Work out the finished part from the listing and answer in its coordinate system (mm). Give positions to 0.01 mm unless a question says otherwise; leave off trailing zeros. Write each loop counter-clockwise with the first axis right and the second up, starting at its lowest first coordinate (ties: lowest second). Pieces come first, ordered by that corner, then holes. Notation, with made-up numbers: (8, -16.5) -> (56, -16.5) arc R27 ccw to (56, 13.5) -> close; hole circle Ø1 at (22, 64). An arc over 180 degrees is marked (long way). Write item = value, one per line. Start each with the question number.
from build123d import *

# Parameters (mm, degrees)
F1_DEPTH = 40
F2_DEPTH = 40
F3_R     = 5


with BuildPart() as f1:
    # F0 (on Top) → F1 (new body)
    with BuildSketch(Plane.XY):
        with BuildLine():
            Line((72.5, 131.3154598667), (72.5, 0))
            ThreePointArc((72.5, 0), (0, -72.5), (-72.5, 0))
            Line((-72.5, 0), (-72.5, 131.3154598667))
            ThreePointArc((-72.5, 131.3154598667), (-131.4940701743, 72.1755464751), (-149.7084414814, -9.3478633504))
            ThreePointArc((-149.7084414814, -9.3478633504), (-138.3891727392, -57.8656795395), (-111.803398875, -100))
            Line((-111.803398875, -100), (0, -100))
            Line((0, -100), (0, -150))
            ThreePointArc((0, -150), (106.066017178, -106.066017178), (150, 0))
            ThreePointArc((150, 0), (129.1801068276, 76.2397534099), (72.5, 131.3154598667))
        make_face()
        with BuildLine():
            ThreePointArc((-72.5, 0), (0, 72.5), (72.5, 0))
            Line((72.5, 0), (72.5, 131.3154598667))
            ThreePointArc((72.5, 131.3154598667), (0, 150), (-72.5, 131.3154598667))
            Line((-72.5, 131.3154598667), (-72.5, 0))
        make_face()
        with BuildLine():
            ThreePointArc((-111.803398875, -100), (-138.3891727392, -57.8656795395), (-149.7084414814, -9.3478633504))
            ThreePointArc((-149.7084414814, -9.3478633504), (-236.0979616676, -71.7417201282), (-338.8482034206, -100))
            Line((-338.8482034206, -100), (-111.803398875, -100))
        make_face()
        with BuildLine():
            Line((-750, -150), (0, -150))
            ThreePointArc((0, -150), (-61.2372435696, -136.9306393763), (-111.803398875, -100))
            Line((-111.803398875, -100), (-338.8482034206, -100))
            Line((-338.8482034206, -100), (-750, -100))
            Line((-750, -100), (-750, -150))
        make_face()
        with BuildLine():
            ThreePointArc((-111.803398875, -100), (-61.2372435696, -136.9306393763), (0, -150))
            Line((0, -150), (0, -100))
            Line((0, -100), (-111.803398875, -100))
        make_face()
    extrude(amount=F1_DEPTH)

    # F0 (on Top) → F2 (cut)
    with BuildSketch(Plane.XY):
        with BuildLine():
            ThreePointArc((-72.5, 0), (0, 72.5), (72.5, 0))
            Line((72.5, 0), (72.5, 131.3154598667))
            ThreePointArc((72.5, 131.3154598667), (0, 150), (-72.5, 131.3154598667))
            Line((-72.5, 131.3154598667), (-72.5, 0))
        make_face()
    extrude(amount=F2_DEPTH, mode=Mode.SUBTRACT)

    # F3
    f3_edges = [f1.edges().sort_by_distance(p)[0] for p in [
        (-750, -150, 20),
        (-72.5, 131.31546, 20),
        (72.5, 131.31546, 20),
        (-750, -100, 20),
    ]]
    fillet(f3_edges, radius=F3_R)


solid = f1.part
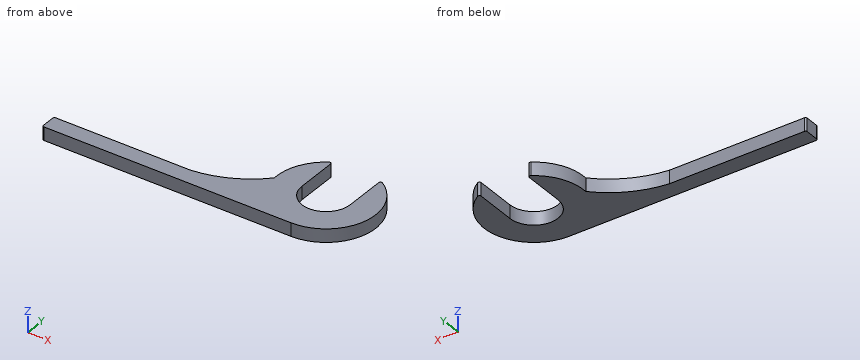
(1) Find the intervals of material crossed by line 1 along X through (y, z) = (3, 11.5); line 2 along X through (y, z) = (7.5, 27.5); line 3 along Y through (x, z) = (-523.5, 22), in increasing order.
(2) Each of these flat-tipped pins is pushed along its axis until it touches: pin 1 (6 mm diameter, centred on x = -42.5, z = 6.5, fed in from +Y); pin 2 (20 mm diameter, centred on y = 55, z = 18, fed in from -X); pin 3 (2 mm diameter, centred on y = -43.5, z = 24.5, fed in from -X). Where does it stop, or does it pass through?
(3) A cutting plane is placed at C-C, the plane y = -63.5. Write down the section's boundary in (x, z).
(4) A cutting plane is placed at B-B, the plane z = 18. Write down the section's boundary in (x, y), then the cut area to 3 significant figures.
(5) A cutting plane is placed at D-D, the plane x = -358. Write down the section's boundary in (y, z), then the cut area to 3 significant figures.
(6) A cutting plane is placed at A-A, the plane y = -30. Write down the section's boundary in (x, z), then the cut area to 3 significant figures.
Results list:
q1.line_1 = -149.97 to -72.5, 72.5 to 149.97
q1.line_2 = -149.81 to -72.5, 72.5 to 149.81
q1.line_3 = -150 to -100
q2.pin_1 = -56.44
q2.pin_2 = -143.09
q2.pin_3 = -190.23
q3.outline = (-220.15, 0) -> (-34.99, 0) -> (-34.99, 40) -> (-220.15, 40) -> close; (34.99, 0) -> (135.9, 0) -> (135.9, 40) -> (34.99, 40) -> close
q4.outline = (-750, -145) arc R5 ccw to (-745, -150) -> (0, -150) arc R150 ccw to (80.17, 126.78) arc R5 ccw to (72.5, 122.55) -> (72.5, 0) arc R72.5 cw to (-72.5, 0) -> (-72.5, 122.55) arc R5 ccw to (-80.17, 126.78) arc R150 ccw to (-149.71, -9.35) arc R300 cw to (-338.85, -100) -> (-745, -100) arc R5 ccw to (-750, -105) -> close
q4.area = 82,200 mm²
q5.outline = (-150, 0) -> (-100, 0) -> (-100, 40) -> (-150, 40) -> close
q5.area = 2,000 mm²
q6.outline = (-171.71, 0) -> (-66, 0) -> (-66, 40) -> (-171.71, 40) -> close; (66, 0) -> (146.97, 0) -> (146.97, 40) -> (66, 40) -> close
q6.area = 7,470 mm²
